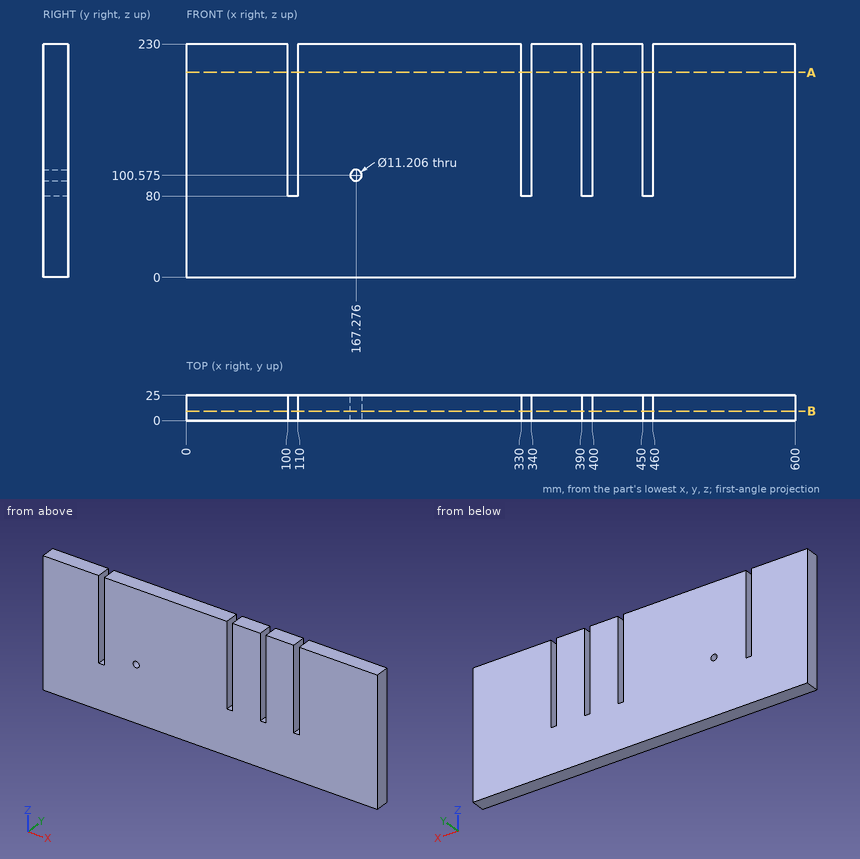
Design review of the part shown in the three views and the two pictorial views. Dimensions are in mm from the part's minimum x, y and z. Coordinates: 2 decimals unless noted, no trailing zeros. Loops run counter-clockwise (first coordinate to the right, second up) from the corner with the lowest first, then second, coordinate; pieces in that order, holes last. Notation, with made-up numbers: (-17.75, -32) -> (6.25, -32) arc R21 ccw to (6.25, 7) -> close; hole circle Ø4 at (72, 12.25). An arc over 180 degrees is marked (long way). Answer as CSV lines item,"result".
Item 1: Insertion check: pin 1 (3 mm diameter, centred on x = 457, y = 12, fed in from +Z). The pin has a flat end and moves straight along its axis. Give the tip position at first contact, or say it passes through.
Results below:
pin 1,"stops at z = 80"
Item 2: Take a section at B-B, the plane y = 9.5. State the section outline as (x, z) points (1 decimal), and give its area (3 significant figures).
Results below:
outline,"(0, 0) -> (600, 0) -> (600, 230) -> (460, 230) -> (460, 80) -> (450, 80) -> (450, 230) -> (400, 230) -> (400, 80) -> (390, 80) -> (390, 230) -> (340, 230) -> (340, 80) -> (330, 80) -> (330, 230) -> (110, 230) -> (110, 80) -> (100, 80) -> (100, 230) -> (0, 230) -> close; hole circle Ø11.2 at (167.3, 100.6)"
area,"132,000 mm2"
Item 3: For L1, parallel to X at y = 8, z = 136; L2, parallel to Z at x = 330.5, y = 8, list the stretches that pass through material, from the lowest coordinate up.
Results below:
L1,"x = 0 to 100, 110 to 330, 340 to 390, 400 to 450, 460 to 600"
L2,"z = 0 to 80"
Item 4: Take a section at A-A, the plane z = 202. State the section outline as (x, y) points, and give its area (3 significant figures).
Results below:
outline,"(0, 0) -> (100, 0) -> (100, 25) -> (0, 25) -> close; (110, 0) -> (330, 0) -> (330, 25) -> (110, 25) -> close; (340, 0) -> (390, 0) -> (390, 25) -> (340, 25) -> close; (400, 0) -> (450, 0) -> (450, 25) -> (400, 25) -> close; (460, 0) -> (600, 0) -> (600, 25) -> (460, 25) -> close"
area,"14,000 mm2"
